Source: CAD feature listing. Evaluate the final solid. Frame: model axes, mm. A direction names the side the tool comes from. Round coordinates to 2 decimals unless told otherwise and drop trailing zeros. Order: outer loops, then holes, each group sorted by start corner. A loop starts at its lowest first (then second) coordinate and runs counter-clockwise, first axis right, second up. Notation, with made-up numbers: (-5.5, 89.25) - (14.5, 89.25) arc R19 ccw to (14.5, 112.25) - close; hole circle Ø3 at (88, 59). An arc over 180 degrees is marked (long way). Return JSON: item names as keys, results as strings. Group by question number.
1) Contact query for a flat-ended pin moving along its axis: P1, Ø1.5, axis at x = 17, y = 19, coming from the +Z side. Output: stop coordinate, or through.
2) Section B-B, the plane y = 18.25. Return loops of the section in (x, z).
3) Section C-C, the plane x = 29.5. Return loops of the section in (y, z).
4) Access query for faces 1 (the flat face through (53, 11, 14)), 2 (the flat face through (56, 11, 13)). Directions: +Z, -Z, +X, -X, +Y, -Y. A direction counts if a zero-diameter tool reaches every point of the face in a straight line with its end or side. Return the directions, or none.
5) Section A-A, the plane z = 9. Return loops of the section in (x, y).
6) Ray query, line 1 (X direction, y = 1.5, z = 13.5); line 2 (Z direction, x = 16, y = 6). Return the intervals inside material, ascending. Write a range as from..to.
```python
from build123d import *

# Parameters (mm, degrees)
BOX_W         = 3
BOX_H         = 23
BOX_DEPTH     = 23
ARRAY_X_COUNT = 2
ARRAY_X_PITCH = 53
BOX001_W      = 56
BOX001_H      = 23
BOX001_DEPTH  = 3


with BuildPart() as baseandtoparray:
    # Box → Box (new body)
    with BuildSketch(Plane.XY.offset(3)):
        with Locations((1.5, 11.5)):
            Rectangle(BOX_W, BOX_H)
    extrude(amount=BOX_DEPTH)

    # Array X: baseAndTopArray ×2


with BuildPart() as baseandtoparray_1:
    add(baseandtoparray.part)
    with Locations(*[(i * ARRAY_X_PITCH, 0, 0) for i in range(1, ARRAY_X_COUNT)]):
        add(baseandtoparray.part)


with BuildPart() as obj1:
    # Box001 → Box001 (new body)
    with BuildSketch(Plane.XY):
        with Locations((28, 11.5)):
            Rectangle(BOX001_W, BOX001_H)
    extrude(amount=BOX001_DEPTH)

    # Fusion: union baseAndTopArray
    add(baseandtoparray_1.part)


solid = obj1.part
```
Geometry check:
{
 "1": {"P1": "z = 3"},
 "2": {"outline": "(0, 0) - (56, 0) - (56, 26) - (53, 26) - (53, 3) - (3, 3) - (3, 26) - (0, 26) - close"},
 "3": {"outline": "(0, 0) - (23, 0) - (23, 3) - (0, 3) - close"},
 "4": {"face 1": "+Z, +Y, -Y", "face 2": "+Z, -Z, +X, +Y, -Y"},
 "5": {"outline": "(0, 0) - (3, 0) - (3, 23) - (0, 23) - close; (53, 0) - (56, 0) - (56, 23) - (53, 23) - close"},
 "6": {"line 1": "0..3, 53..56", "line 2": "0..3"}
}
